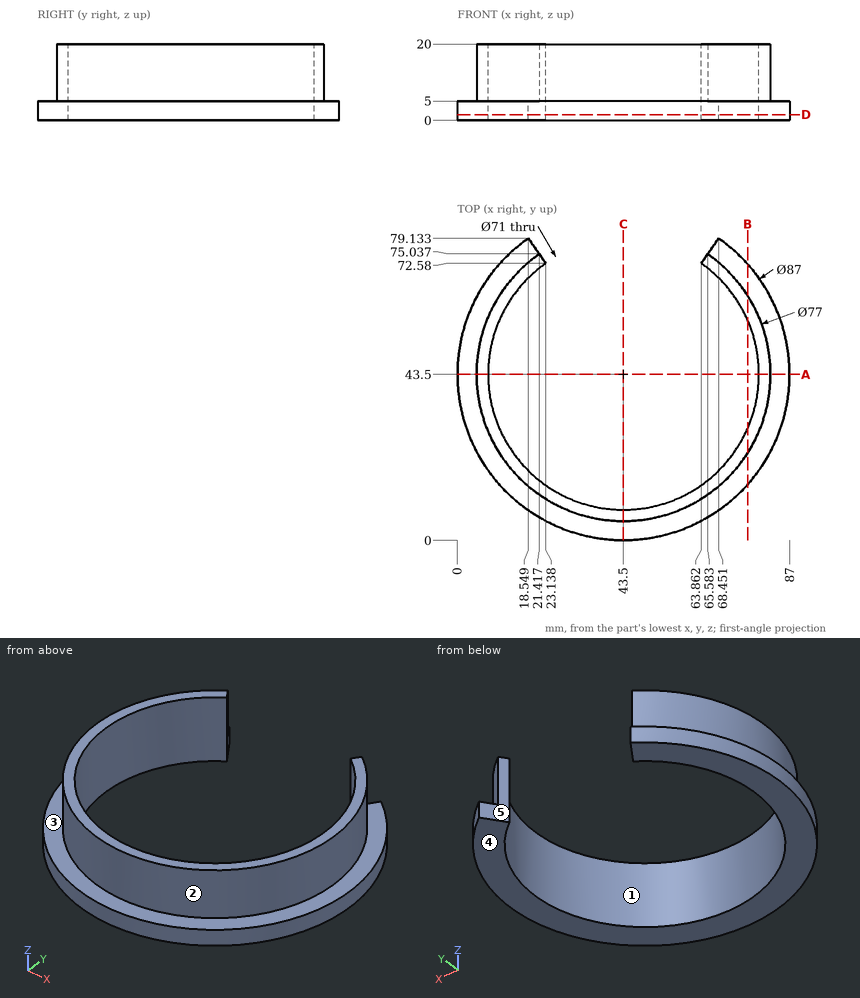
Check sheet for the drawn part. Datum: minimum x, y, z corner. Units: mm. A direction names the side the tool comes from. Round coordinates to 2 decimals unless told otherwise and drop trailing zeros. Order: outer loops, then holes, each group sorted by start corner. A loop starts at its lowest first (then second) coordinate and runs counter-clockwise, first axis right, second up. Notation, with made-up numbers: (87, 45) -> (134, 45) arc R21 ccw to (134, 71) -> close; hole circle Ø4 at (55, 84). An arc over 180 degrees is marked (long way). Put each result on its own line as item: value.
1) Section check B-B (x = 76). Record the cut outline in (y, z).
Final values:
outline: (14.59, 0) -> (29.22, 0) -> (29.22, 20) -> (22.86, 20) -> (22.86, 5) -> (14.59, 5) -> close; (57.78, 0) -> (72.41, 0) -> (72.41, 5) -> (64.14, 5) -> (64.14, 20) -> (57.78, 20) -> close
2) Mould release check, pull along X, two halves, no side actions. Record for the marked faces 1, 2 and 3: +X half, -X half, draft (parallel to the pull), parting line (faces both ways), or undercut.
Final values:
face 1: undercut
face 2: parting line
face 3: draft
3) Depth check by flat-ended pin: pin 1 (3 mm diameter, centred on x = 34, z = 11, fed in from +Y); pin 2 (1.5 mm diameter, centred on y = 10.5, z = 4, fed in from -X); pin 3 (4 mm diameter, centred on x = 9, z = 9.5, fed in from +Y). Enter the tip coordinate at first touch or a pass-through.
Final values:
pin 1: stops at y = 9.75
pin 2: stops at x = 14.31
pin 3: stops at y = 64.14
4) Set-up check for the marked faces 4 and 5: record each of +Z, -Z, +X, -X, +Y, -Y from which the full face is reachable in a straight line by a thin tool's end or side.
Final values:
face 4: -Z, +X, -X, +Y, -Y
face 5: +Z, -Z, +Y
5) Section check D-D (z = 1.5). Record the cut outline in (x, y).
Final values:
outline: (18.55, 79.13) arc R43.5 ccw (long way) to (68.45, 79.13) -> (63.86, 72.58) arc R35.5 cw (long way) to (23.14, 72.58) -> close
6) Material ranges on line 1 (X direction, y = 43.5, z = 10); line 2 (X direction, y = 65.5, z = 7.25) (1 decimal); line 3 (Z direction, x = 8.5, y = 60.5), recorded low to high.
Final values:
line 1: x = 5 to 8, 79 to 82
line 2: x = 11.9 to 15.6, 71.4 to 75.1
line 3: z = 0 to 5
7) Section check C-C (x = 43.5). Record the cut outline in (y, z).
Final values:
outline: (0, 0) -> (8, 0) -> (8, 20) -> (5, 20) -> (5, 5) -> (0, 5) -> close
8) Section check A-A (y = 43.5). Record the cut outline in (x, z), then the cut area to 3 significant figures.
Final values:
outline: (0, 0) -> (8, 0) -> (8, 20) -> (5, 20) -> (5, 5) -> (0, 5) -> close; (79, 0) -> (87, 0) -> (87, 5) -> (82, 5) -> (82, 20) -> (79, 20) -> close
area: 170 mm^2
